Source: CAD feature listing. Evaluate the final solid. Frame: model axes, mm. Face numbers are marked on the shaded views. A direction names the side the tool comes from. Round coordinates to 2 decimals unless told otherwise and drop trailing zeros. Order: outer loops, then holes, each group sorted by start corner. A loop starts at its lowest first (then second) coordinate and runs counter-clockwise, first axis right, second up. Notation, with made-up numbers: (61.5, 73.5) - (118.5, 73.5) arc R26 cw to (118.5, 104.5) - close; hole circle Ø3 at (79, 7.5). An arc over 180 degrees is marked (long way). Put each result on its own line as item: value. Start each with the question number.
1) Section D-D on x = -15.5. Output: boundary loops of the cut face in (y, z).
2) Section B-B on x = 36.5. Output: boundary loops of the cut face in (y, z).
3) Line query: probe 1 along Y at (x, z) = (36.5, 5.5); probe 2 along Y at (x, z) = (7.5, 9.5); probe 3 along X at (y, z) = (35, 10) (3 decimals). Output: solid intervals per line, ascending. Write a range as [from, to].
4) Section A-A on y = 33.5. Output: boundary loops of the cut face in (x, z) (3 decimals), then the cut area to 3 significant figures.
5) Mould query, pull axis X, two halves, no side actions, for the marked faces 1, 2, 3 and 4. Classes: +X half, -X half, draft (parallel to the pull), parting line (faces both ways), or undercut.
6) Contact query for flat-ended pins moving along their axis: P1, Ø8, axis at y = -20, z = 9.5, coming from the -X side (3 decimals); P2, Ø12, axis at x = 16, y = 19, coming from the +Z side; P3, Ø9.5, axis at y = -19, z = 8.5, coming from the +X side (3 decimals). Output: stop coordinate, or through.
7) Access query for the marked faces 5, 6, 7, 8 and 9. Directions: +Z, -Z, +X, -X, +Y, -Y. A direction counts if a zero-diameter tool reaches every point of the face in a straight line with its end or side. Return the directions, or none.
8) Section C-C on z = 9.5. Output: boundary loops of the cut face in (x, y) (3 decimals), then the cut area to 3 significant figures.
```python
from build123d import *

# Parameters (mm, degrees)
SKETCH_1_W               = 79.25
SKETCH_1_H               = 62.72
EXTRUDE_1_DEPTH          = 19
SKETCH_2_W               = 69.25
SKETCH_2_H               = 52.72
CUT_EXTRUDE_1_DEPTH      = 16
CUT_EXTRUDE_2_DEPTH      = 10
CUT_EXTRUDE_3_DEPTH      = 77.582889897
CUT_EXTRUDE_3_DEPTH_BACK = 77.582889897
SKETCH_4_R               = 1.5
EXTRUDE_START            = -55
SKETCH_5_R               = 1.7
EXTRUDE_2_DEPTH          = 10
SKETCH_6_R               = 3
CUT_EXTRUDE_4_DEPTH      = 3


with BuildPart() as part:
    # 草图1 → 凸台-拉伸1 (new body)
    with BuildSketch(Plane.XY):
        with Locations((0, 31.36)):
            Rectangle(SKETCH_1_W, SKETCH_1_H)
    extrude(amount=EXTRUDE_1_DEPTH)

    # 草图2 → 切除-拉伸1 (cut)
    with BuildSketch(Plane.XY.offset(19)):
        with Locations((0, 31.36)):
            Rectangle(SKETCH_2_W, SKETCH_2_H)
    extrude(amount=-CUT_EXTRUDE_1_DEPTH, mode=Mode.SUBTRACT)

    # 草图3 → 切除-拉伸2 (cut)
    with BuildSketch(Plane(origin=(0, 0, 0), x_dir=(-1, 0, 0), z_dir=(0, 0, -1))):
        Polygon((12.5, 40), (-12.5, 40), (-12.5, 23), (-22.5, 23), (-22.5, 8), (22.5, 8), (22.5, 23), (12.5, 23), align=None)
    extrude(amount=-CUT_EXTRUDE_2_DEPTH, mode=Mode.SUBTRACT)

    # 草图4 → 切除-拉伸3 (cut, two sides: drawn at the far end of the back side and taken through both)
    with BuildSketch(Plane(origin=(0, 0, 0), x_dir=(-1, 0, 0), z_dir=(0, 0, -1)).offset(-CUT_EXTRUDE_3_DEPTH_BACK)):
        with Locations((-36.5, 59.72)):
            Circle(SKETCH_4_R)
        with Locations(Location((36.5, 59.72, 0), (0, 0, 180))):
            Circle(SKETCH_4_R)
        with Locations(Location((-36.5, 3, 0), (0, 0, 180))):
            Circle(SKETCH_4_R)
        with Locations((36.5, 3)):
            Circle(SKETCH_4_R)
    extrude(amount=CUT_EXTRUDE_3_DEPTH + CUT_EXTRUDE_3_DEPTH_BACK, mode=Mode.SUBTRACT)

    # 草图5 → 凸台-拉伸2 (add)
    with BuildSketch(Plane.ZY.offset(39.625).offset(EXTRUDE_START)):
        with BuildLine():
            Line((0, 0), (0, -20))
            ThreePointArc((0, -20), (9.5, -29.5), (19, -20))
            Line((19, -20), (19, 0))
            Line((19, 0), (0, 0))
        make_face()
        with Locations(Location((9.5, -20, 0), (0, 0, 270))):
            Circle(SKETCH_5_R, mode=Mode.SUBTRACT)
    extrude(amount=EXTRUDE_2_DEPTH)

    # 草图6 → 切除-拉伸4 (cut)
    with BuildSketch(Plane(origin=(15.375, 0, 0), x_dir=(0, 0, -1), z_dir=(1, 0, 0))):
        with Locations(Location((-9.5, -20, 0), (0, 0, 90))):
            Circle(SKETCH_6_R)
    extrude(amount=-CUT_EXTRUDE_4_DEPTH, mode=Mode.SUBTRACT)


solid = part.part
```
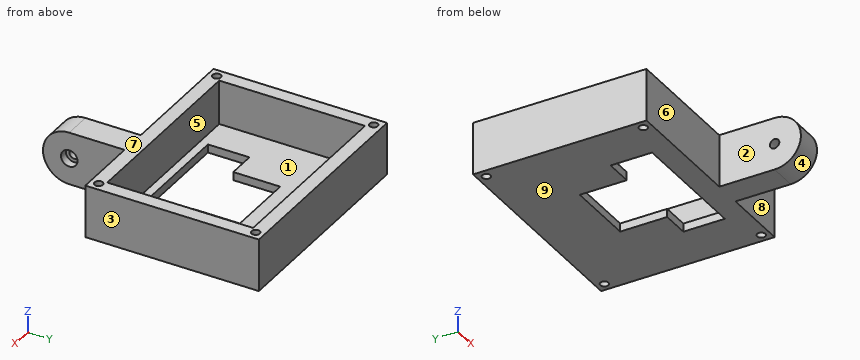
Answer sheet:
1. outline: (0, 0) - (8, 0) - (8, 3) - (5, 3) - (5, 19) - (0, 19) - close; (23, 0) - (62.72, 0) - (62.72, 19) - (57.72, 19) - (57.72, 3) - (23, 3) - close
2. outline: (0, 0) - (1.5, 0) - (1.5, 19) - (0, 19) - close; (4.5, 0) - (58.22, 0) - (58.22, 19) - (4.5, 19) - close; (61.22, 0) - (62.72, 0) - (62.72, 19) - (61.22, 19) - close
3. probe 1: [0, 1.5], [4.5, 58.22], [61.22, 62.72]
3. probe 2: [-29.5, -21.7], [-18.3, 5], [57.72, 62.72]
3. probe 3: [-39.625, -34.625], [34.625, 39.625]
4. outline: (-39.625, 0) - (-12.5, 0) - (-12.5, 3) - (-34.625, 3) - (-34.625, 19) - (-39.625, 19) - close; (12.5, 0) - (39.625, 0) - (39.625, 19) - (34.625, 19) - (34.625, 3) - (12.5, 3) - close
4. area: 323 mm^2
5. face 1: undercut
5. face 2: -X half
5. face 3: +X half
5. face 4: draft
6. P1: x = 5.375
6. P2: z = 3
6. P3: x = 15.375
7. face 5: +Z
7. face 6: +Z, -Z, -X, -Y
7. face 7: +Z, +X, -X, +Y, -Y
7. face 8: +Z, -Z, +X, -Y
7. face 9: -Z, +X, -X, +Y, -Y
8. outline: (-39.625, 0) - (5.375, 0) - (5.375, -18.3) - (12.375, -18.3) - (12.375, -17) - (15.375, -17) - (15.375, 0) - (39.625, 0) - (39.625, 62.72) - (-39.625, 62.72) - close; (5.375, -29.5) - (15.375, -29.5) - (15.375, -23) - (12.375, -23) - (12.375, -21.7) - (5.375, -21.7) - close; hole circle Ø3 at (-36.5, 3); hole circle Ø3 at (-36.5, 59.72); hole (-34.625, 5) - (34.625, 5) - (34.625, 57.72) - (-34.625, 57.72) - close; hole circle Ø3 at (36.5, 3); hole circle Ø3 at (36.5, 59.72)
8. area: 1,540 mm^2
